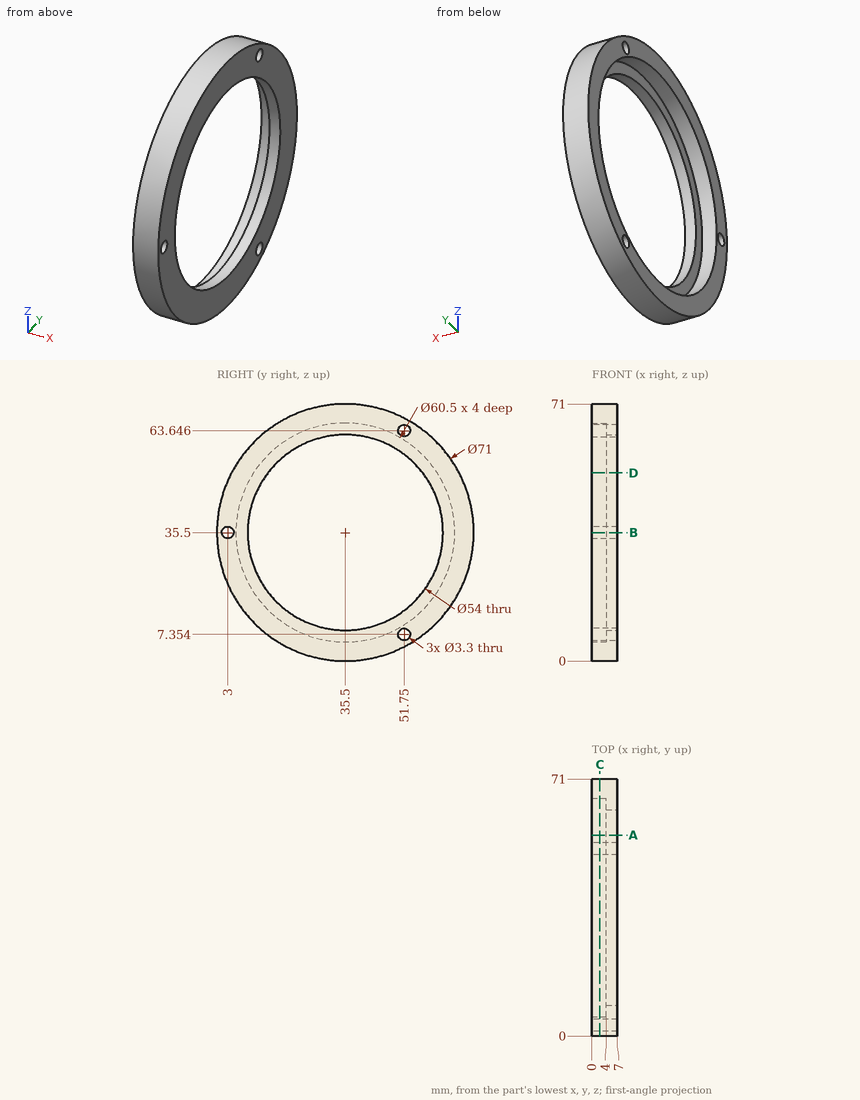
Print and shaded views of the part. All mm, measured from the part's lowest x, y and z. Round coordinates to 2 decimals unless told otherwise and drop trailing zeros. Write each loop counter-clockwise with the first axis right and the second up, starting at its lowest first coordinate (ties: lowest second). Pieces come first, ordered by that corner, then holes. Notation, with made-up numbers: (52, -14) -> (82, -14) arc R19 cw to (82, 3) -> close; hole circle Ø6 at (54, 12.25). An arc over 180 degrees is marked (long way). Write item = value, one per line.
(1) Band-saw the part on A-A (y = 55.5). Give the cut face in (x, z) (1 decimal).
Answer:
outline = (0, 6.2) -> (7, 6.2) -> (7, 17.4) -> (4, 17.4) -> (4, 12.8) -> (0, 12.8) -> close; (0, 58.2) -> (4, 58.2) -> (4, 53.6) -> (7, 53.6) -> (7, 64.8) -> (0, 64.8) -> close
(2) Flat gauge pins, fed straight in: pin 1 (2 mm diameter, centred on x = 3, z = 53.5, fed in from +Y) (1 decimal); pin 2 (1.5 mm diameter, centred on x = 2, y = 45, fed in from +Z) (1 decimal). Where does each tip first touch, or does it go through?
Answer:
pin_1 = 66.7
pin_2 = 69.9
(3) Band-saw the part on C-C (x = 2.25). Give the cut face in (y, z).
Answer:
outline = circle Ø71 at (35.5, 35.5); hole circle Ø3.3 at (3, 35.5); hole circle Ø60.5 at (35.5, 35.5); hole circle Ø3.3 at (51.75, 7.35); hole circle Ø3.3 at (51.75, 63.65)
(4) Band-saw the part on D-D (z = 52). Give the cut face in (x, y), then the cut area to 3 significant figures.
Answer:
outline = (0, 4.07) -> (7, 4.07) -> (7, 14.13) -> (4, 14.13) -> (4, 10.15) -> (0, 10.15) -> close; (0, 60.85) -> (4, 60.85) -> (4, 56.87) -> (7, 56.87) -> (7, 66.93) -> (0, 66.93) -> close
area = 109 mm2
(5) Band-saw the part on B-B (z = 35.5). Give the cut face in (x, y), then the cut area to 3 significant figures.
Answer:
outline = (0, 0) -> (7, 0) -> (7, 1.35) -> (0, 1.35) -> close; (0, 4.65) -> (7, 4.65) -> (7, 8.5) -> (4, 8.5) -> (4, 5.25) -> (0, 5.25) -> close; (0, 65.75) -> (4, 65.75) -> (4, 62.5) -> (7, 62.5) -> (7, 71) -> (0, 71) -> close
area = 69.9 mm2
(6) Probe L1, parallel to Y at x = 3, z = 35.5; L2, parallel to X at y = 6, z = 35; L3, parallel to Z at x = 1.75, y = 51.75 (1 decimal). List the from-to ranges inside material, lowest first.
Answer:
L1 = 0 to 1.35, 4.65 to 5.25, 65.75 to 71
L2 = 4 to 7
L3 = 3.9 to 5.7, 9 to 10, 61 to 62, 65.3 to 67.1
